from build123d import *

# Parameters (mm, degrees)
F0_W     = 50
F0_H     = 33
F0_R     = 2
F0_R_2   = 1
F1_DEPTH = 7
F2_W     = 50
F2_H     = 18
F2_R     = 1
F2_R_2   = 2
F3_DEPTH = 15


with BuildPart() as f1:
    # F0 (on Front) → F1 (new body)
    with BuildSketch(Plane.XZ):
        with Locations((25, -16.5)):
            Rectangle(F0_W, F0_H)
        with Locations((7.5, -18.5)):
            Circle(F0_R, mode=Mode.SUBTRACT)
        with Locations((19.5, -24)):
            Circle(F0_R_2, mode=Mode.SUBTRACT)
        with Locations((28.5, -24)):
            Circle(F0_R_2, mode=Mode.SUBTRACT)
        with Locations((42.5, -5.5)):
            Circle(F0_R, mode=Mode.SUBTRACT)
    extrude(amount=F1_DEPTH)

    # F2 (on Front) → F3 (join)
    with BuildSketch(Plane.XZ):
        with Locations((25, -24)):
            Rectangle(F2_W, F2_H)
        with Locations((19.5, -24)):
            Circle(F2_R, mode=Mode.SUBTRACT)
        with Locations((7.5, -18.5)):
            Circle(F2_R_2, mode=Mode.SUBTRACT)
        with Locations((28.5, -24)):
            Circle(F2_R, mode=Mode.SUBTRACT)
    extrude(amount=F3_DEPTH)


solid = f1.part
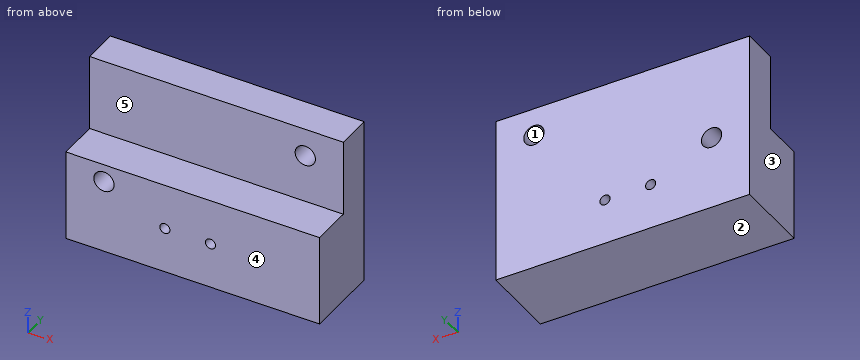
The model under review builds one solid part; all positions refer to its coordinate system, in mm. Face numbers are marked on the shaded views. A direction names the side the tool comes from. Give positions to 0.01 mm unless a question says otherwise; leave off trailing zeros. Order: outer loops, then holes, each group sorted by start corner. A loop starts at its lowest first (then second) coordinate and runs counter-clockwise, first axis right, second up. Notation, with made-up numbers: (68, 9.5) -> (95, 9.5) arc R34 cw to (95, 48.5) -> close; hole circle Ø8 at (-10, 9.5). An arc over 180 degrees is marked (long way). Write item = value, one per line. Start each with the question number.
(1) Draft analysis for pull direction Z (two halves, no side actions). For the marked faces 1, 2 and 3, state which applies: +Z half, -Z half, draft (parallel to the pull), parting line (faces both ways), or undercut.
(2) Tool access review of the marked faces 4 and 5: name each direction out of +Z, -Z, +X, -X, +Y, -Y from which nothing blocks a thin tool from reaching the whole face with its end or side.
(3) Take a section at C-C (y = -13.25). Write out the cut boundary in (x, z).
(4) Take a section at A-A (z = -5.5). Write out the cut boundary in (x, y), plus the area to 3 significant figures.
(5) Take a section at B-B (x = 19.5). Write out the cut boundary in (y, z).
(6) For pin 1 Ø1.5 at (x, z) = (42, -14) entering from -Y, flat-tipped, find the tip position at first contact; note if it passes through.
(7) For L1, parallel to Z at x = 28.5, y = -8.75; L2, parallel to Z at x = 7.5, y = -5.25; L3, parallel to Z at x = 38.5, y = -14, list the stretches that pass through material, from the lowest coordinate up. Write a range as from..to.
(8) Take a section at D-D (y = -2.5). Write out the cut boundary in (x, z).
Returned:
q1.face_1 = undercut
q1.face_2 = -Z half
q1.face_3 = draft
q2.face_4 = +Z, -Z, +X, -X, -Y
q2.face_5 = +Z, +X, -X, -Y
q3.outline = (0, -33) -> (50, -33) -> (50, -15) -> (0, -15) -> close; hole circle Ø4 at (7.5, -18.5); hole circle Ø2 at (19.5, -24); hole circle Ø2 at (28.5, -24)
q4.outline = (0, -7) -> (40.5, -7) -> (40.5, 0) -> (0, 0) -> close; (44.5, -7) -> (50, -7) -> (50, 0) -> (44.5, 0) -> close
q4.area = 322 mm²
q5.outline = (-15, -33) -> (0, -33) -> (0, -25) -> (-15, -25) -> close; (-15, -23) -> (0, -23) -> (0, 0) -> (-7, 0) -> (-7, -15) -> (-15, -15) -> close
q6.pin_1 = -7
q7.L1 = -33..-25, -23..-15
q7.L2 = -33..-20.5, -16.5..0
q7.L3 = -33..-15
q8.outline = (0, -33) -> (50, -33) -> (50, 0) -> (0, 0) -> close; hole circle Ø4 at (7.5, -18.5); hole circle Ø2 at (19.5, -24); hole circle Ø2 at (28.5, -24); hole circle Ø4 at (42.5, -5.5)
